Answer from the drawing. Dimensions are ordinates in mm from the lowest x, y and z of the part. A direction names the side the tool comes from. Coordinates: 2 decimals unless noted, no trailing zeros. Order: outer loops, then holes, each group sorted by start corner. A loop starts at its lowest first (then second) coordinate and runs counter-clockwise, first axis right, second up.
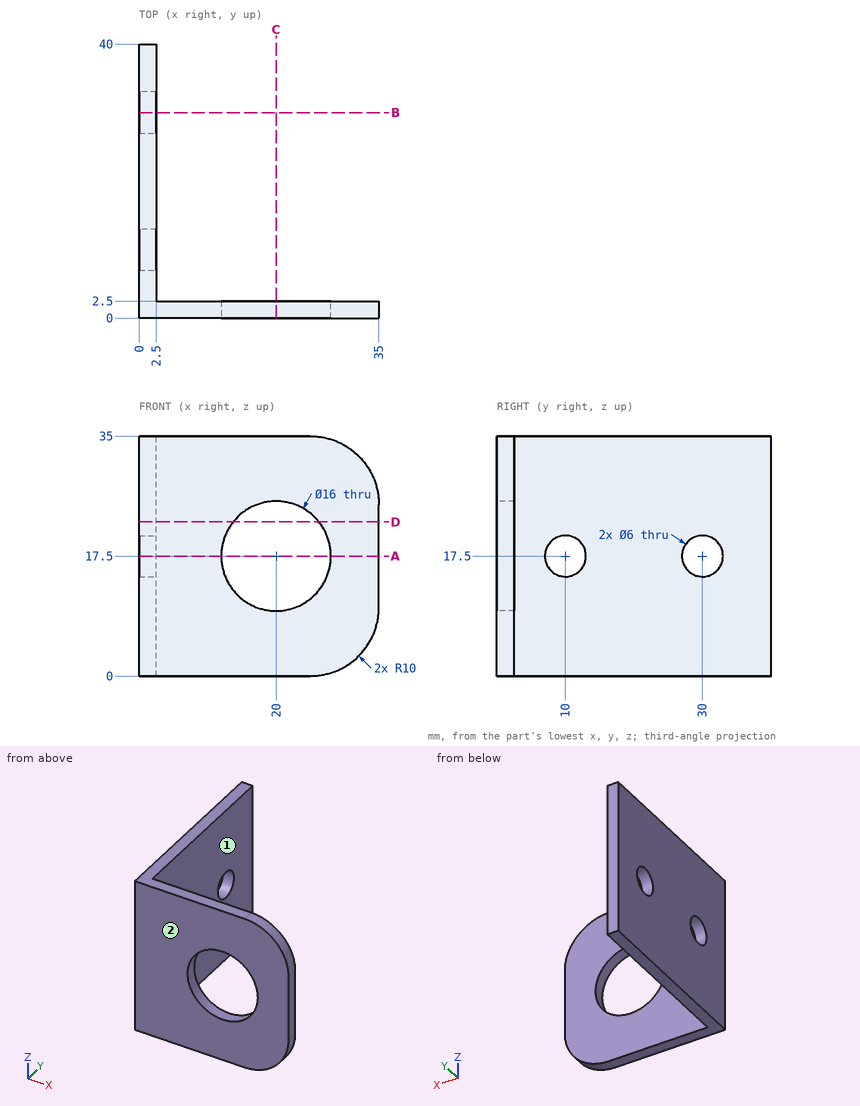
1. The part is cut by section B-B (y = 30). Determine the outline of the cut face in (x, z), plus the area to 3 significant figures.
2. Flat-ended cylindrical pins translate along their axes: pin 1 (7 mm diameter, centred on y = 30, z = 17.5, fed in from +X); pin 2 (16 mm diameter, centred on x = 22, z = 15, fed in from +Y). Find the tip coordinate at first contact, or state that the pin passes through.
3. The part is cut by section C-C (x = 20). Determine the outline of the cut face in (y, z).
4. The part is cut by section D-D (z = 22.5). Determine the outline of the cut face in (x, y) (3 decimals), plus the area to 3 significant figures.
5. The part is cut by section A-A (z = 17.5). Determine the outline of the cut face in (x, y).
6. Consider probe 1 along Z at (x, y) = (20, 1.6); probe 2 along Z at (x, y) = (1.85, 10); probe 3 along Y at (x, z) = (1, 17). Determine where each line is inside the solid, lowest interval first.
7. For the marked faces 1 and 2, determine the directions among +Z, -Z, +X, -X, +Y, -Y from which every point of the face is accessible in a straight line to the end or side of a thin tool.
Worked out:
1. outline: (0, 0) - (2.5, 0) - (2.5, 14.5) - (0, 14.5) - close; (0, 20.5) - (2.5, 20.5) - (2.5, 35) - (0, 35) - close
1. area: 72.5 mm2
2. pin 1: stops at x = 2.5
2. pin 2: stops at y = 2.5
3. outline: (0, 0) - (2.5, 0) - (2.5, 9.5) - (0, 9.5) - close; (0, 25.5) - (2.5, 25.5) - (2.5, 35) - (0, 35) - close
4. outline: (0, 0) - (13.755, 0) - (13.755, 2.5) - (2.5, 2.5) - (2.5, 40) - (0, 40) - close; (26.245, 0) - (35, 0) - (35, 2.5) - (26.245, 2.5) - close
4. area: 150 mm2
5. outline: (0, 0) - (12, 0) - (12, 2.5) - (2.5, 2.5) - (2.5, 7) - (0, 7) - close; (0, 13) - (2.5, 13) - (2.5, 27) - (0, 27) - close; (0, 33) - (2.5, 33) - (2.5, 40) - (0, 40) - close; (28, 0) - (35, 0) - (35, 2.5) - (28, 2.5) - close
6. probe 1: z = 0 to 9.5, 25.5 to 35
6. probe 2: z = 0 to 14.5, 20.5 to 35
6. probe 3: y = 0 to 7.04, 12.96 to 27.04, 32.96 to 40
7. face 1: +Z, -Z, +X, +Y
7. face 2: +Z, -Z, +X, -X, -Y
